from build123d import *

# Parameters (mm, degrees)
F0_R      = 1.65
F1_DEPTH  = 4
F2_W      = 6
F2_H      = 14.7
F2_W_2    = 16
F2_H_2    = 6
F3_DEPTH  = 4
F4_W      = 6
F4_H      = 6
F5_DEPTH  = 20
F6_DEPTH  = 1.5
F7_DEPTH  = 11
F8_R      = 1.65
F9_DEPTH  = 14.701
F10_R     = 1.35
F11_DEPTH = 80.001
F12_R     = 1.35
F13_DEPTH = 65.001
F14_R     = 2.99999
F15_R     = 1.35
F16_DEPTH = 24.001


# Not quite as in the source:
# - a fillet or chamfer is up to 0.001 mm smaller than in the source, because OpenCascade refuses the exact size


with BuildPart() as f1:
    # F0 (on Front) → F1 (new body)
    with BuildSketch(Plane.XZ):
        Polygon((-25, 6.3), (-40, 6.3), (-40, -4.3), (-40, -19), (-34, -19), (-34, -4.3), (-8, -4.3), (-8, -10.3), (8, -10.3), (8, -4.3), (34, -4.3), (34, -19), (40, -19), (40, -4.3), (40, 6.3), (25, 6.3), (25, 12.3), (19, 12.3), (19, 6.3), (-19, 6.3), (-19, 12.3), (-25, 12.3), align=None)
        with Locations((-37, 0)):
            Circle(F0_R, mode=Mode.SUBTRACT)
        with Locations((37, 0)):
            Circle(F0_R, mode=Mode.SUBTRACT)
    extrude(amount=F1_DEPTH)

    # F2 (on face) → F3 (join)
    with BuildSketch(Plane(origin=(0, 0, 0), x_dir=(-1, 0, 0), z_dir=(0, 1, 0))):
        with Locations((37, -11.65)):
            Rectangle(F2_W, F2_H)
        with Locations((0, -7.3)):
            Rectangle(F2_W_2, F2_H_2)
        with Locations((-37, -11.65)):
            Rectangle(F2_W, F2_H)
    extrude(amount=F3_DEPTH)

    # F4 (on face) → F5 (join)
    with BuildSketch(Plane(origin=(0, 0, 0), x_dir=(-1, 0, 0), z_dir=(0, 1, 0))):
        with Locations((-22, 9.3)):
            Rectangle(F4_W, F4_H)
        with Locations((22, 9.3)):
            Rectangle(F4_W, F4_H)
    extrude(amount=F5_DEPTH)

    # F6 (add): faces of the model
    f6_faces = [f1.faces().sort_by_distance(p)[0] for p in [
        (22, 10, 6.3),
        (-22, 10, 6.3),
    ]]
    extrude(f6_faces, amount=F6_DEPTH)

    # F7 (add): a face of the model
    f7_faces = [f1.faces().sort_by_distance(p)[0] for p in [
        (0, 4, -7.3),
    ]]
    extrude(f7_faces, amount=F7_DEPTH)

    # F8 (on face) → F9 (cut, through all)
    with BuildSketch(Plane.XY.offset(-4.3)):
        with Locations((5, 12)):
            Circle(F8_R)
        with Locations((-5, 12)):
            Circle(F8_R)
    extrude(amount=-F9_DEPTH, mode=Mode.SUBTRACT)

    # F10 (on face) → F11 (cut, through all)
    with BuildSketch(Plane.YZ.offset(40)):
        with Locations((0, -15)):
            Circle(F10_R)
    extrude(amount=-F11_DEPTH, mode=Mode.SUBTRACT)

    # F12 (on face) → F13 (cut, through all)
    with BuildSketch(Plane(origin=(-25, 0, 0), x_dir=(0, -1, 0), z_dir=(-1, 0, 0))):
        with Locations((-16.25, 8.55)):
            Circle(F12_R)
    extrude(amount=-F13_DEPTH, mode=Mode.SUBTRACT)

    # F14 (radius 3 in the source; OpenCascade refuses exactly that, so slightly less here)
    f14_edges = [f1.edges().sort_by_distance(p)[0] for p in [
        (-37, -4, -19),
        (37, -4, -19),
        (37, 4, -19),
        (-37, 4, -19),
        (8, 15, -7.3),
        (-8, 15, -7.3),
        (-22, 20, 12.3),
        (22, 20, 12.3),
        (-22, 20, 4.8),
        (22, 20, 4.8),
        (-22, -4, 12.3),
        (22, -4, 12.3),
        (-34, -2, -4.3),
        (34, -2, -4.3),
        (-8, -2, -4.3),
        (8, -2, -4.3),
        (-25, -2, 6.3),
        (19, -2, 6.3),
        (-19, -2, 6.3),
        (25, -2, 6.3),
        (-40, -2, 6.3),
        (40, -2, 6.3),
        (0, -4, -10.3),
    ]]
    fillet(f14_edges, radius=F14_R)

    # F15 (on face) → F16 (cut, through all)
    with BuildSketch(Plane.XZ.offset(4)):
        with Locations((-20, 0)):
            Circle(F15_R)
        with Locations((20, 0)):
            Circle(F15_R)
    extrude(amount=-F16_DEPTH, mode=Mode.SUBTRACT)


solid = f1.part
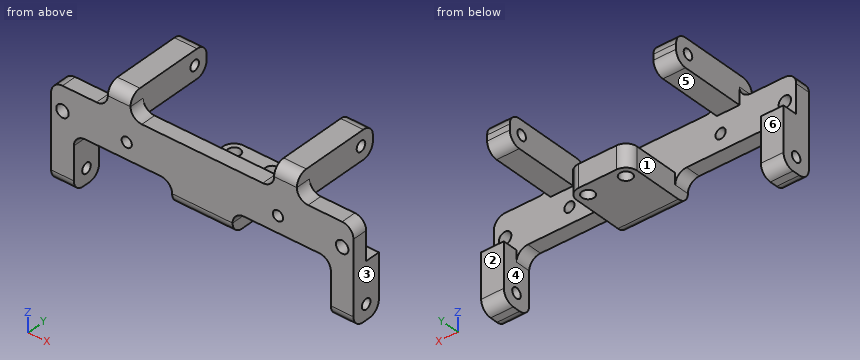
Verification items for the finished model (mm, model axes). Face numbers are marked on the shaded views. A direction names the side the tool comes from. Coordinates: 2 decimals unless noted, no trailing zeros. Order: outer loops, then holes, each group sorted by start corner. A loop starts at its lowest first (then second) coordinate and runs counter-clockwise, first axis right, second up. Notation, with made-up numbers: M 11,64 L 28,64 A9 cw 28,72 Z; hole C 70.5,7.5 d8. An arc over 180 degrees is marked long. One line per item, written item: value. Start each with the question number.
Item 1: Sectioned sample at D-D on z = 8.55. Record the cut outline in (x, y), then the cut area to 3 significant figures.
Item 2: Mould release check, pull along X, two halves, no side actions. Record for the marked faces 1, 2 and 3: pulls with the +X half, pulls with the -X half, needs draft (parallel to the pull), parting line crosses it, or undercut.
Item 3: Depth check by flat-ended pin: P1, Ø1, axis at x = 2, y = 1, coming from the +Z side; P2, Ø6, axis at y = 11, z = 7.5, coming from the -X side; P3, Ø8, axis at y = 3.5, z = 9.5, coming from the +X side. Enter the tip coordinate at first touch or a pass-through.
Item 4: Sectioned sample at A-A on y = 7. Record the cut outline in (x, z).
Item 5: Sectioned sample at B-B on x = 20. Record the cut outline in (y, z), then the cut area to 3 significant figures.
Item 6: Sectioned sample at C-C on y = 16.25. Record the cut outline in (x, z), then the cut area to 3 significant figures.
Item 7: Thickness scan on probe 1 along X at (y, z) = (3.25, -9); probe 2 along X at (y, z) = (14.75, 5); probe 3 along Y at (x, z) = (5, -5). Record the ranges inside material, lowest first.
Item 8: Access from +Z, -Z, +X, -X, +Y, -Y to the whole of each face (thin tool, end or side, straight path). Record for the marked faces 4, 5 and 6.
Calculated:
1. outline: M -25.1,-4 L -18.9,-4 L -18.9,0 L -19,0 L -19,14.9 L -25,14.9 L -25,0 L -25.1,0 Z; M -25,17.6 L -19,17.6 L -19,20 L -25,20 Z; M 18.9,-4 L 25.1,-4 L 25.1,0 L 25,0 L 25,14.9 L 19,14.9 L 19,0 L 18.9,0 Z; M 19,17.6 L 25,17.6 L 25,20 L 19,20 Z
1. area: 257 mm^2
2. face 1: undercut
2. face 2: needs draft
2. face 3: pulls with the +X half
3. P1: z = -4.3
3. P2: x = -25
3. P3: x = 25.55
4. outline: M -25,4.8 L -19,4.8 L -19,12.3 L -25,12.3 Z; M -8,-10.3 L 8,-10.3 L 8,-4.3 L -8,-4.3 Z; M 19,4.8 L 25,4.8 L 25,12.3 L 19,12.3 Z
5. outline: M -4,-4.3 L 0,-4.3 L 0,-1.35 L -4,-1.35 Z; M -4,1.35 L 0,1.35 L 0,4.8 L 17,4.8 A3 ccw 20,7.8 L 20,9.3 A3 ccw 17,12.3 L -1,12.3 A3 ccw -4,9.3 Z; hole C 16.25,8.55 d2.7
5. area: 194 mm^2
6. outline: M -25,4.8 L -19,4.8 L -19,7.2 L -25,7.2 Z; M -25,9.9 L -19,9.9 L -19,12.3 L -25,12.3 Z; M 19,4.8 L 25,4.8 L 25,7.2 L 19,7.2 Z; M 19,9.9 L 25,9.9 L 25,12.3 L 19,12.3 Z
6. area: 57.6 mm^2
7. probe 1: -40 to -34, -8 to 8, 34 to 40
7. probe 2: -25 to -19, 19 to 25
7. probe 3: -4 to 10.35, 13.65 to 15
8. face 4: -Z, +Y
8. face 5: -Z, +X, -X, +Y
8. face 6: +Z, -Z, -X, +Y
